Input: part model. Units: mm. Frame: model coordinates. Face numbers are marked on the shaded views. A direction names the side the tool comes from. Round coordinates to 2 decimals unless told otherwise and drop trailing zeros. Loops run counter-clockwise (first coordinate to the right, second up) from the corner with the lowest first, then second, coordinate; pieces in that order, holes last. Notation, with made-up numbers: (-5, -27.5) -> (16, -27.5) arc R27 ccw to (16, 9.5) -> close; hole circle Ø10 at (-8, 33.5). An arc over 180 degrees is marked (long way). Answer in a Markdown table with one row per item. Add a question column.
Q1. Section B-B, the plane x = 10.75. Output: boundary loops of the cut face in (y, z).
Q2. Pin query (flat end, axial travel): pin 1 (3 mm diameter, centred on y = 38.5, z = 10.5, fed in from -X); pin 2 (6 mm diameter, centred on x = 7, y = 20.5, fed in from -Z); pin 3 (3 mm diameter, centred on x = 16, z = 9, fed in from -Y); pin 4 (3 mm diameter, centred on x = 10, y = 4, fed in from +Z). Return the tip coordinate at first contact, or that it passes through.
Q3. Reachability of the marked faces 1, 2, 3 and 4 from +Z, -Z, +X, -X, +Y, -Y: full face, straight path, thin tool, end or side. Return the list, or none.
Q4. Ray query, L1, parallel to Y at x = 20, z = 11; L2, parallel to Y at x = 11.25, z = 4.75; L3, parallel to Y at x = 7, z = 14. Return the intervals inside material, ascending. Write a range as from..to.
Q5. Section D-D, the plane x = 2.5. Output: boundary loops of the cut face in (y, z).
Q6. Mould query, pull axis Y, two halves, no side actions, for the marked faces 5, 6 and 7. Classes: pulls with the +Y half, pulls with the -Y half, needs draft (parallel to the pull), parting line crosses it, or undercut.
Q7. Section A-A, the plane z = 11.75. Output: boundary loops of the cut face in (x, y), and give its area (3 significant figures).
Q8. Section C-C, the plane y = 16.5. Output: boundary loops of the cut face in (x, z).
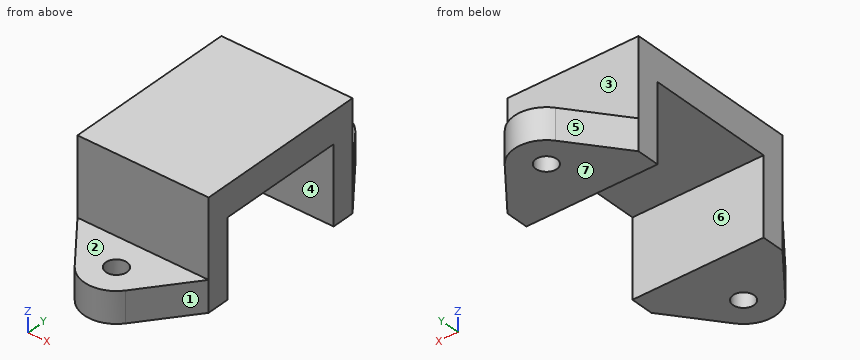
```python
from build123d import *

# Parameters (mm, degrees)
SKETCH5_R             = 1.7
BOSS_EXTRUDE5_DEPTH   = 5
BOSS_EXTRUDE5_2_DEPTH = 5
SKETCH6_W             = 21.205551353
SKETCH6_H             = 3.684327219
BOSS_EXTRUDE6_DEPTH   = 7.5
SKETCH7_W             = 21.205551353
SKETCH7_H             = 28.068654438
BOSS_EXTRUDE7_DEPTH   = 5


with BuildPart() as part:
    # Sketch5 → Boss-Extrude5 (new body)
    with BuildSketch(Plane.XY):
        with BuildLine():
            Line((7.492385077, 44.529251739), (1, 36.146663352))
            Line((1, 36.146663352), (1, 32.462336133))
            Line((1, 32.462336133), (5.2, 32.462336133))
            Line((5.2, 32.462336133), (22.205551353, 32.462336133))
            Line((22.205551353, 32.462336133), (22.205551353, 36.146663352))
            Line((22.205551353, 36.146663352), (15.713166275, 44.529251739))
            ThreePointArc((15.713166275, 44.529251739), (11.602775676, 46.544776073), (7.492385077, 44.529251739))
        make_face()
        with Locations((11.602775676, 41.345719713)):
            Circle(SKETCH5_R, mode=Mode.SUBTRACT)
    extrude(amount=BOSS_EXTRUDE5_DEPTH)



with BuildPart() as body_2:
    # Sketch5 → Boss-Extrude5 2 (new body)
    with BuildSketch(Plane.XY):
        with BuildLine():
            Line((5.2, 11.762336133), (1, 11.762336133))
            Line((1, 11.762336133), (1, 8.078008914))
            Line((1, 8.078008914), (7.492385077, -0.304579472))
            ThreePointArc((7.492385077, -0.304579472), (11.602775676, -2.320103807), (15.713166275, -0.304579472))
            Line((15.713166275, -0.304579472), (22.205551353, 8.078008914))
            Line((22.205551353, 8.078008914), (22.205551353, 11.762336133))
            Line((22.205551353, 11.762336133), (5.2, 11.762336133))
        make_face()
        with Locations((11.602775676, 2.878952554)):
            Circle(SKETCH5_R, mode=Mode.SUBTRACT)
    extrude(amount=BOSS_EXTRUDE5_2_DEPTH)


with BuildPart() as part_1:
    add(part.part)

    add(body_2.part)  # Boss-Extrude6 merges body 2
    # Sketch6 → Boss-Extrude6 (add)
    with BuildSketch(Plane.XY.offset(5)):
        with Locations((11.602775677, 9.920172523)):
            Rectangle(SKETCH6_W, SKETCH6_H)
        with Locations((11.602775677, 34.304499742)):
            Rectangle(SKETCH6_W, SKETCH6_H)
    extrude(amount=BOSS_EXTRUDE6_DEPTH)

    # Sketch7 → Boss-Extrude7 (add)
    with BuildSketch(Plane.XY.offset(12.5)):
        with Locations((11.602775677, 22.112336133)):
            Rectangle(SKETCH7_W, SKETCH7_H)
    extrude(amount=BOSS_EXTRUDE7_DEPTH)


solid = part_1.part
```
Answer block:
| question | item | result |
|---|---|---|
| 1 | outline | (-2.25, 0) -> (1.41, 0) -> (1.41, 5) -> (-2.25, 5) -> close; (4.35, 0) -> (11.76, 0) -> (11.76, 12.5) -> (32.46, 12.5) -> (32.46, 0) -> (39.88, 0) -> (39.88, 5) -> (36.15, 5) -> (36.15, 17.5) -> (8.08, 17.5) -> (8.08, 5) -> (4.35, 5) -> close; (42.82, 0) -> (46.47, 0) -> (46.47, 5) -> (42.82, 5) -> close |
| 2 | pin 1 | through |
| 2 | pin 2 | z = 12.5 |
| 2 | pin 3 | y = 8.08 |
| 2 | pin 4 | z = 5 |
| 3 | face 1 | +Z, -Z, +X, -Y |
| 3 | face 2 | +Z, +X, -X, -Y |
| 3 | face 3 | +Z, +X, -X, +Y |
| 3 | face 4 | -Z, +X, -X |
| 4 | L1 | 8.08..11.76, 32.46..36.15 |
| 4 | L2 | -2.31..1.22, 4.54..11.76, 32.46..39.68, 43.01..46.53 |
| 4 | L3 | 8.08..36.15 |
| 5 | outline | (6.14, 0) -> (11.76, 0) -> (11.76, 12.5) -> (32.46, 12.5) -> (32.46, 0) -> (38.08, 0) -> (38.08, 5) -> (36.15, 5) -> (36.15, 17.5) -> (8.08, 17.5) -> (8.08, 5) -> (6.14, 5) -> close |
| 6 | face 5 | pulls with the +Y half |
| 6 | face 6 | undercut |
| 6 | face 7 | needs draft |
| 7 | outline | (1, 8.08) -> (22.21, 8.08) -> (22.21, 11.76) -> (1, 11.76) -> close; (1, 32.46) -> (22.21, 32.46) -> (22.21, 36.15) -> (1, 36.15) -> close |
| 7 | area | 156 mm^2 |
| 8 | outline | (1, 12.5) -> (22.21, 12.5) -> (22.21, 17.5) -> (1, 17.5) -> close |
